Check sheet for the drawn part. Datum: minimum x, y, z corner. Units: mm. Round coordinates to 2 decimals unless told otherwise and drop trailing zeros. Write each loop counter-clockwise with the first axis right and the second up, starting at its lowest first coordinate (ties: lowest second). Pieces come first, ordered by that corner, then holes. Notation, with made-up numbers: M -2.75,-3 L 42.25,-3 A23 cw 42.25,20 Z; hole C 20.25,-22 d6. An arc over 180 degrees is marked long. One line per item, written item: value. Start each with the question number.
Item 1: Section check C-C, the plane y = 217. Record the cut outline in (x, z), then the cut area to 3 significant figures.
Item 2: Thickness scan on probe 1 along Y at (x, z) = (40.5, 6.5); probe 2 along X at (y, z) = (197.5, 2.75). Record the ranges inside material, lowest first. Write a range as from..to.
Item 3: Gauge pin test, flat ends, axial feed: pin 1 (5 mm diameter, centred on x = 30.5, z = 7, fed in from +Y); pin 2 (3 mm diameter, centred on y = 36.5, z = 6.5, fed in from +X). Record the tip position at first contact, or that the pin passes through.
Item 4: Section check B-B, the plane z = 7.5. Record the cut outline in (x, y), then the cut area to 3 significant figures.
Item 5: Section check A-A, the plane x = 20. Record the cut outline in (y, z), then the cut area to 3 significant figures.
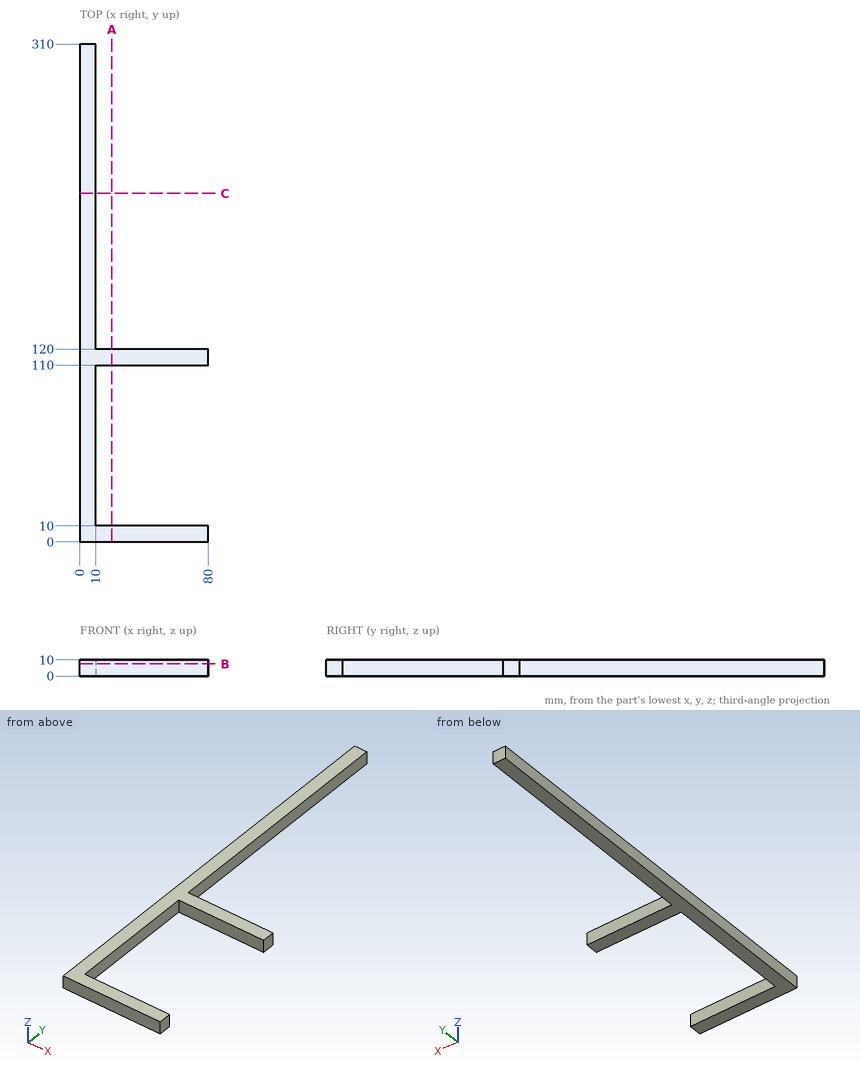
Response values:
1. outline: M 0,0 L 10,0 L 10,10 L 0,10 Z
1. area: 100 mm2
2. probe 1: y = 0..10, 110..120
2. probe 2: x = 0..10
3. pin 1: stops at y = 120
3. pin 2: stops at x = 10
4. outline: M 0,0 L 80,0 L 80,10 L 10,10 L 10,110 L 80,110 L 80,120 L 10,120 L 10,310 L 0,310 Z
4. area: 4,500 mm2
5. outline: M 0,0 L 10,0 L 10,10 L 0,10 Z; M 110,0 L 120,0 L 120,10 L 110,10 Z
5. area: 200 mm2
